from build123d import *

# Parameters (mm, degrees)
BOSS_EXTRUDE1_DEPTH = 2
BOSS_EXTRUDE2_DEPTH = 20
BOSS_EXTRUDE3_DEPTH = 23
CHAMFER1_SIZE       = 1
CUT_EXTRUDE1_DEPTH  = 28
CUT_EXTRUDE2_DEPTH  = 19
CHAMFER2_SIZE       = 1
BOSS_EXTRUDE4_START = 5
BOSS_EXTRUDE4_DEPTH = 2
SKETCH8_R           = 1.5
CUT_EXTRUDE3_DEPTH  = 2
SKETCH9_R           = 1.625
CUT_EXTRUDE4_DEPTH  = 5
SKETCH10_R          = 1.25
BOSS_EXTRUDE5_DEPTH = 2


with BuildPart() as part:
    # Sketch2 → Boss-Extrude1 (new body)
    with BuildSketch(Plane.XY):
        Polygon((29.88488863, -2.595574528), (29.88488863, -26.295574528), (17.64488863, -26.295574528), (17.64488863, -38.295574528), (54.12488863, -38.295574528), (54.12488863, -26.295574528), (41.88488863, -26.295574528), (41.88488863, -2.595574528), align=None)
    extrude(amount=BOSS_EXTRUDE1_DEPTH)

    # Sketch3 → Boss-Extrude2 (add)
    with BuildSketch(Plane(origin=(0, 0, 0), x_dir=(-1, 0, 0), z_dir=(0, 0, -1))):
        Polygon((-53.12488863, -37.295574528), (-53.12488863, -27.295574528), (-41.12488863, -27.295574528), (-36.12488863, -32.295574528), (-41.12488863, -37.295574528), align=None)
        Polygon((-35.64488863, -32.295574528), (-30.64488863, -27.295574528), (-18.64488863, -27.295574528), (-18.64488863, -37.295574528), (-30.64488863, -37.295574528), align=None)
    extrude(amount=BOSS_EXTRUDE2_DEPTH)

    # Sketch3<3> → Boss-Extrude3 (add)
    with BuildSketch(Plane(origin=(0, 0, 0), x_dir=(-1, 0, 0), z_dir=(0, 0, -1))):
        Polygon((-40.88488863, -3.595574528), (-30.88488863, -3.595574528), (-30.88488863, -23.557914395), (-35.88488863, -28.557914395), (-40.88488863, -23.557914395), align=None)
    extrude(amount=BOSS_EXTRUDE3_DEPTH)

    # Chamfer1
    chamfer1_edges = [part.edges().sort_by_distance(p)[0] for p in [
        (53.12488863, -32.295574528, -20),
        (47.12488863, -37.295574528, -20),
        (38.62488863, -34.795574528, -20),
        (38.62488863, -29.795574528, -20),
        (47.12488863, -27.295574528, -20),
        (33.14488863, -29.795574528, -20),
        (33.14488863, -34.795574528, -20),
        (24.64488863, -37.295574528, -20),
        (18.64488863, -32.295574528, -20),
        (24.64488863, -27.295574528, -20),
        (40.88488863, -13.576744462, -23),
        (38.38488863, -26.057914395, -23),
        (33.38488863, -26.057914395, -23),
        (30.88488863, -13.576744462, -23),
        (35.88488863, -3.595574528, -23),
    ]]
    chamfer(chamfer1_edges, length=CHAMFER1_SIZE)

    # Sketch4 → Cut-Extrude1 (cut)
    with BuildSketch(Plane.XY.offset(2)):
        Polygon((31.88488863, -23.338741615), (31.88488863, -4.595574528), (39.88488863, -4.595574528), (39.88488863, -23.338741615), (35.88488863, -27.338741615), align=None)
    extrude(amount=-CUT_EXTRUDE1_DEPTH, mode=Mode.SUBTRACT)

    # Sketch4<3> → Cut-Extrude2 (cut)
    with BuildSketch(Plane.XY.offset(2)):
        Polygon((19.64488863, -36.312819682), (19.64488863, -28.295574528), (29.88488863, -28.295574528), (33.88488863, -32.295574528), (29.867643476, -36.312819682), align=None)
        Polygon((37.88488863, -32.295574528), (41.88488863, -28.295574528), (52.12488863, -28.295574528), (52.12488863, -36.295574528), (41.88488863, -36.295574528), align=None)
    extrude(amount=-CUT_EXTRUDE2_DEPTH, mode=Mode.SUBTRACT)

    # Chamfer2
    chamfer2_edges = [part.edges().sort_by_distance(p)[0] for p in [
        (19.64488863, -32.304197105, -17),
        (24.76488863, -28.295574528, -17),
        (31.88488863, -30.295574528, -17),
        (31.876266053, -34.304197105, -17),
        (24.756266053, -36.312819682, -17),
        (39.88488863, -30.295574528, -17),
        (47.00488863, -28.295574528, -17),
        (52.12488863, -32.295574528, -17),
        (47.00488863, -36.295574528, -17),
        (39.88488863, -34.295574528, -17),
    ]]
    chamfer(chamfer2_edges, length=CHAMFER2_SIZE)

    # Sketch7 → Boss-Extrude4 (add)
    with BuildSketch(Plane(origin=(0, 0, 0), x_dir=(-1, 0, 0), z_dir=(0, 0, -1)).offset(BOSS_EXTRUDE4_START)):
        with BuildLine():
            Line((-30.88488863, -9.295574528), (-30.88488863, -27.295574528))
            Line((-30.88488863, -27.295574528), (-20.930717386, -27.295574528))
            add(Edge.make_bspline(
                [(-20.930717386, -27.295574528), (-20.930717386, -9.295574528), (-30.88488863, -9.295574528)],
                knots=[4.71238898, 4.71238898, 4.71238898, 6.283185307, 6.283185307, 6.283185307], degree=2, weights=[1, 0.707106781, 1]))
        make_face()
        with BuildLine():
            Line((-40.88488863, -27.295574528), (-50.839059874, -27.295574528))
            add(Edge.make_bspline(
                [(-40.88488863, -9.295574528), (-50.839059874, -9.295574528), (-50.839059874, -27.295574528)],
                knots=[0, 0, 0, 1.570796327, 1.570796327, 1.570796327], degree=2, weights=[1, 0.707106781, 1]))
            Line((-40.88488863, -9.295574528), (-40.88488863, -27.295574528))
        make_face()
    extrude(amount=BOSS_EXTRUDE4_DEPTH)

    # Sketch8 → Cut-Extrude3 (cut)
    with BuildSketch(Plane(origin=(0, 0, -7), x_dir=(-1, 0, 0), z_dir=(0, 0, -1))):
        with Locations((-25.71892105, -18.498352077)):
            Circle(SKETCH8_R)
        with Locations(Location((-46.05085621, -18.498352077, 0), (0, 0, 180))):
            Circle(SKETCH8_R)
    extrude(amount=-CUT_EXTRUDE3_DEPTH, mode=Mode.SUBTRACT)

    # Sketch9 → Cut-Extrude4 (cut)
    with BuildSketch(Plane.XZ.offset(37.295574528)):
        with Locations(Location((23.88488863, -13.628778028, 0), (0, 0, 270))):
            Circle(SKETCH9_R)
        with Locations(Location((47.88488863, -13.628778028, 0), (0, 0, 270))):
            Circle(SKETCH9_R)
    extrude(amount=-CUT_EXTRUDE4_DEPTH, mode=Mode.SUBTRACT)

    # Sketch10 → Boss-Extrude5 (add)
    with BuildSketch(Plane.XY.offset(-17)):
        with Locations((46.906421739, -32.180011543)):
            Circle(SKETCH10_R)
        with Locations((24.906421739, -32.180011543)):
            Circle(SKETCH10_R)
    extrude(amount=BOSS_EXTRUDE5_DEPTH)


solid = part.part
Geometry: final body of the model. Coordinates: model frame, mm. A direction names the side the tool comes from. Coordinates: 2 decimals unless noted, no trailing zeros. Order: outer loops, then holes, each group sorted by start corner. A loop starts at its lowest first (then second) coordinate and runs counter-clockwise, first axis right, second up.
1) Section C-C (x = 35). Return loops of the section in (y, z), then the cut area to 3 significant figures.
Result sheet:
outline: (-38.3, 0) - (-32.94, 0) - (-32.94, -19) - (-32.3, -19.46) - (-31.65, -19) - (-31.65, 0) - (-27.67, 0) - (-27.67, -22) - (-26.45, -22.86) - (-26.45, 2) - (-38.3, 2) - close; (-4.6, -23) - (-3.6, -22) - (-3.6, 0) - (-2.6, 0) - (-2.6, 2) - (-4.6, 2) - close
area: 102 mm2
2) Section B-B (y = -7.5). Return loops of the section in (x, z), then the cut area to 3 significant figures.
Result sheet:
outline: (29.88, 0) - (30.88, 0) - (30.88, -22) - (31.88, -23) - (31.88, 2) - (29.88, 2) - close; (39.88, -23) - (40.88, -22) - (40.88, 0) - (41.88, 0) - (41.88, 2) - (39.88, 2) - close
area: 53.0 mm2
3) Set-up query: faces 4 (the flat face through (24.828, -35.806, -16.507)), 5 (the flat face through (41.885, -15, 1)), 6 (the flat face through (38.59, -34.76, -9.37)), 7 (the flat face through (47, -27.296, -9)). Return all of +Z, -Z, +X, -X, +Y, -Y with unobstructed straight access to the full face (end or side cutting, diameter ignored); none if empty.
Result sheet:
face 4: +Z
face 5: +Z, +X, +Y
face 6: -Z, -Y
face 7: +X, +Y
4) Draft query along Z for faces 1 (the flat face through (39.02, -30.12, -19.51)), 2 (the flat face through (20.152, -32.36, -16.507)), 3 (the cylindrical face through (22.299, -36.811, -13.277)). Return one class per face: released by +Z, released by -Z, zero draft, split by the parting line, or undercut.
Result sheet:
face 1: released by -Z
face 2: released by +Z
face 3: undercut
5) First-contact query: P1, Ø6, axis at y = -10, z = -15, coming from the +X side; P2, Ø1.6, axis at x = 45, z = 1.5, coming from the +Y side; P3, Ø13, axis at x = 25.5, z = -7, coming from the -Y side; P4, Ø2, axis at x = 26.5, y = -7.5, coming from the -Z side. Flat tips, straight axial feed; report the tip coordinate or a pass-through.
Result sheet:
P1: stops at x = 40.88
P2: stops at y = -26.3
P3: stops at y = -37.3
P4: passes through
6) Ray query, probe 1 along X at (y, z) = (-5.5, -16); probe 2 along Y at (x, z) = (29, -16); probe 3 along Y at (x, z) = (25, -16.25). Return the intervals inside material, ascending.
Result sheet:
probe 1: x = 30.88 to 31.88, 39.88 to 40.88
probe 2: y = -37.3 to -36.31, -28.3 to -27.3
probe 3: y = -37.3 to -36.06, -33.43 to -30.93, -28.55 to -27.3
7) Section A-A (z = -4). Give the number of separate pieces and of enclosed holes in the cut face, then the cut area to 3 significant figures.
Result sheet:
separate pieces: 3
enclosed holes: 3
area: 153 mm2
